from build123d import *

# Parameters (mm, degrees)
SKETCH1_W           = 480
SKETCH1_H           = 315
BOSS_EXTRUDE1_DEPTH = 330
SKETCH9_W           = 460
SKETCH9_H           = 300
CUT_EXTRUDE1_DEPTH  = 320
CHAMFER1_SIZE       = 30
CHAMFER2_SIZE       = 30
SKETCH11_W          = 360
SKETCH11_H          = 10
BOSS_EXTRUDE2_DEPTH = 20
SKETCH12_W          = 360
SKETCH12_H          = 8
BOSS_EXTRUDE3_DEPTH = 60
FILLET1_R           = 10


with BuildPart() as part:
    # Sketch1 → Boss-Extrude1 (new body)
    with BuildSketch(Plane(origin=(0, 0, 0), x_dir=(1, 0, 0), z_dir=(0, 1, 0))):
        Rectangle(SKETCH1_W, SKETCH1_H)
    extrude(amount=BOSS_EXTRUDE1_DEPTH)

    # Sketch9 → Cut-Extrude1 (cut)
    with BuildSketch(Plane(origin=(0, 330, 0), x_dir=(1, 0, 0), z_dir=(0, 1, 0))):
        Rectangle(SKETCH9_W, SKETCH9_H)
    extrude(amount=-CUT_EXTRUDE1_DEPTH, mode=Mode.SUBTRACT)

    # Chamfer1
    chamfer1_edges = [part.edges().sort_by_distance(p)[0] for p in [
        (230, 170, -150),
        (230, 170, 150),
        (-230, 170, 150),
        (-230, 170, -150),
        (-240, 165, -157.5),
        (240, 165, -157.5),
        (240, 165, 157.5),
        (-240, 165, 157.5),
    ]]
    chamfer(chamfer1_edges, length=CHAMFER1_SIZE)

    # Chamfer2
    chamfer2_edges = [part.edges().sort_by_distance(p)[0] for p in [
        (0, 0, -157.5),
        (-240, 0, 0),
        (240, 0, 0),
        (0, 0, 157.5),
        (225, 0, 142.5),
        (-225, 0, 142.5),
        (-225, 0, -142.5),
        (225, 0, -142.5),
        (230, 10, 0),
        (0, 10, 150),
        (0, 10, -150),
        (-230, 10, 0),
        (215, 10, -135),
        (-215, 10, -135),
        (-215, 10, 135),
        (215, 10, 135),
    ]]
    chamfer(chamfer2_edges, length=CHAMFER2_SIZE)

    # Sketch11 → Boss-Extrude2 (add)
    with BuildSketch(Plane.XY.offset(157.5)):
        with Locations((0, 235.251091022)):
            Rectangle(SKETCH11_W, SKETCH11_H)
    extrude(amount=BOSS_EXTRUDE2_DEPTH)

    # Sketch12 → Boss-Extrude3 (add)
    with BuildSketch(Plane.XZ.offset(-230.251091022)):
        with Locations((0, 173.5)):
            Rectangle(SKETCH12_W, SKETCH12_H)
    extrude(amount=BOSS_EXTRUDE3_DEPTH)

    # Fillet1
    # the kernel refuses this fillet: 10 mm, written as the material it takes off along each edge
    with BuildSketch(Plane(origin=(-204.494897428, 170.251091022, 177.5), x_dir=(0, 0, -1), z_dir=(1, 0, 0))) as fillet1_piece_1:
        with BuildLine():
            CenterArc((10, 9.797958971), FILLET1_R, 180, 78.463040967)
            Line((0, 9.797958971), (-0.2, 9.797958971))
            Line((-0.2, 9.797958971), (-0.2, 0))
            Line((-0.2, 0), (0, -0.2))
            ThreePointArc((0, -0.2), (4, -0.2), (7.96, -0.195959179))
            Line((7.96, -0.195959179), (8, 0))
        make_face()
    extrude(amount=408.989794856, mode=Mode.SUBTRACT)
    with BuildSketch(Plane(origin=(205, 240.251091022, 177.5), x_dir=(0, -1, 0), z_dir=(-1, 0, 0))) as fillet1_piece_2:
        with BuildLine():
            CenterArc((FILLET1_R, -FILLET1_R), FILLET1_R, 90, 90)
            Line((0, -FILLET1_R), (-FILLET1_R * 0.02, -FILLET1_R))
            Line((-FILLET1_R * 0.02, -FILLET1_R), (-FILLET1_R * 0.02, FILLET1_R * 0.02))
            Line((-FILLET1_R * 0.02, FILLET1_R * 0.02), (FILLET1_R, FILLET1_R * 0.02))
            Line((FILLET1_R, FILLET1_R * 0.02), (FILLET1_R, 0))
        make_face()
    extrude(amount=410, mode=Mode.SUBTRACT)


solid = part.part
Geometry check sheet. Reference: the model listing, model coordinates, mm. A direction names the side the tool comes from. Round coordinates to 2 decimals unless told otherwise and drop trailing zeros. Loops run counter-clockwise (first coordinate to the right, second up) from the corner with the lowest first, then second, coordinate; pieces in that order, holes last. Notation, with made-up numbers: (-37, -6) - (-22, -6) arc R26 cw to (-22, 11) - close; hole circle Ø4 at (13.25, -9). An arc over 180 degrees is marked (long way). Answer as CSV lines item,"result".
(1) Cross-section at D-D, the plane z = 143.5. Enter the section's corners in (x, y), and give its area (3 significant figures).
Output values:
outline,"(-224, 30) - (-204.2, 16) - (204.2, 16) - (224, 30) - (224, 330) - (206.5, 330) - (206.5, 40) - (197.31, 33.5) - (-197.31, 33.5) - (-206.5, 40) - (-206.5, 330) - (-224, 330) - close"
area,"18,000 mm²"
(2) Cross-section at B-B, the plane x = 37. Enter the section's corners in (y, z).
Output values:
outline,"(0, -127.5) - (30, -157.5) - (330, -157.5) - (330, -150) - (40, -150) - (10, -120) - (10, 120) - (40, 150) - (330, 150) - (330, 157.5) - (240.25, 157.5) - (240.25, 167.5) arc R10 ccw to (230.25, 177.5) - (180.05, 177.5) arc R10 ccw to (170.25, 169.5) - (230.25, 169.5) - (230.25, 157.5) - (30, 157.5) - (0, 127.5) - close"
(3) Release check for a two-part mould opening along X. For faces 4 (the face through (-230, 187, 2)), 5 (the face through (216.689, 18.543, 134.609)), 6 (the face through (-180, 214, 172)) record: released by +X, released by -X, zero draft, split by the parting line, or undercut.
Output values:
face 4,"undercut"
face 5,"released by +X"
face 6,"released by -X"
(4) Material ranges on line 1 along X through (y, z) = (226.5, -49.5); line 2 along Z through (x, y) = (182, 175.5); line 3 along Y through (x, z) = (-145, 69.5), recorded low to high.
Output values:
line 1,"x = -240 to -230, 230 to 240"
line 2,"z = -157.5 to -150, 150 to 157.5"
line 3,"y = 0 to 10"
(5) Depth check by flat-ended pin: pin 1 Ø2 at (x, z) = (-100, 92.5) entering from +Y; pin 2 Ø10 at (y, z) = (211, 171) entering from +X; pin 3 Ø4 at (x, y) = (-133.5, 77.5) entering from +Z. Enter the tip coordinate at first touch or a pass-through.
Output values:
pin 1,"stops at y = 10"
pin 2,"stops at x = 180"
pin 3,"stops at z = 157.5"
(6) Cross-section at A-A, the plane y = 247.5. Enter the section's corners in (x, z).
Output values:
outline,"(-240, -127.5) - (-210, -157.5) - (210, -157.5) - (240, -127.5) - (240, 127.5) - (210, 157.5) - (-210, 157.5) - (-240, 127.5) - close; hole (-230, -120) - (-200, -150) - (200, -150) - (230, -120) - (230, 120) - (200, 150) - (-200, 150) - (-230, 120) - close"
(7) Cross-section at C-C, the plane z = -78. Enter the section's corners in (x, y).
Output values:
outline,"(-240, 30) - (-210, 0) - (210, 0) - (240, 30) - (240, 330) - (230, 330) - (230, 40) - (200, 10) - (-200, 10) - (-230, 40) - (-230, 330) - (-240, 330) - close"
(8) Set-up check for faces 1 (the face through (-3, 230.251, 163)), 2 (the face through (216.689, 18.543, -134.609)), 3 (the face through (-3, 187, -150)): record each of +Z, -Z, +X, -X, +Y, -Y from which the full face is reachable in a straight line by a thin tool's end or side.
Output values:
face 1,"+X, -X, -Y"
face 2,"-Z, +X, -Y"
face 3,"+Y"
